The model under review builds one solid part; all positions refer to its coordinate system, in mm. Face numbers are marked on the shaded views. A direction names the side the tool comes from. Give positions to 0.01 mm unless a question says otherwise; leave off trailing zeros. Write each loop counter-clockwise with the first axis right and the second up, starting at its lowest first coordinate (ties: lowest second). Pieces come first, ordered by that corner, then holes. Notation, with made-up numbers: (76.25, 14) -> (124.25, 14) arc R20 ccw to (124.25, 22) -> close; hole circle Ø1 at (41.25, -17). An arc over 180 degrees is marked (long way). Use CSV: the item, a comma, the result in double quotes.
```python
from build123d import *

# Parameters (mm, degrees)
SKETCH1_R           = 13
SKETCH1_R_2         = 4.5
BOSS_EXTRUDE1_DEPTH = 2
SKETCH1_3_R         = 7
SKETCH1_3_R_2       = 4.5
BOSS_EXTRUDE2_DEPTH = 5
CHAMFER1_SIZE       = 1


with BuildPart() as part:
    # Sketch1 → Boss-Extrude1 (new body)
    with BuildSketch(Plane.XY):
        Circle(SKETCH1_R)
        Circle(SKETCH1_R_2, mode=Mode.SUBTRACT)
    extrude(amount=BOSS_EXTRUDE1_DEPTH)

    # Sketch1<3> → Boss-Extrude2 (add)
    with BuildSketch(Plane.XY):
        Circle(SKETCH1_3_R)
        Circle(SKETCH1_3_R_2, mode=Mode.SUBTRACT)
    extrude(amount=BOSS_EXTRUDE2_DEPTH)

    # Chamfer1
    chamfer1_edges = [part.edges().sort_by_distance(p)[0] for p in [
        (-7, 0, 5),
    ]]
    chamfer(chamfer1_edges, length=CHAMFER1_SIZE)


solid = part.part
```
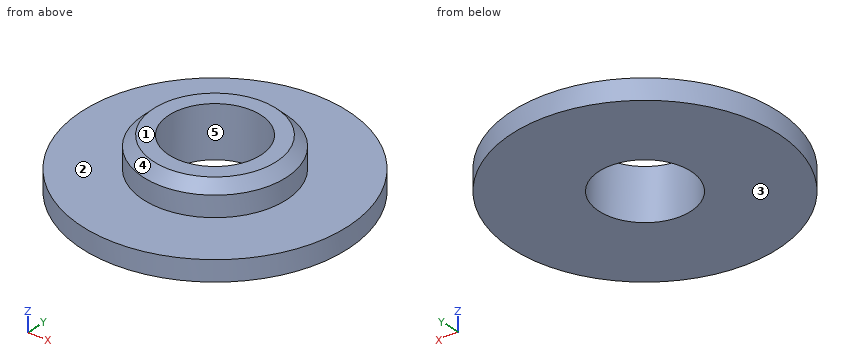
Q1. The part is to be moulded in two halves that separate along Y. For the marked faces 3, 4 and 5, say which applies: pulls with the +Y half, pulls with the -Y half, needs draft (parallel to the pull), parting line crosses it, or undercut.
Derived:
face 3,"needs draft"
face 4,"parting line crosses it"
face 5,"undercut"
Q2. Consider section A-A (x = 0). Write out the cut boundary in (y, z).
Derived:
outline,"(-13, 0) -> (-4.5, 0) -> (-4.5, 5) -> (-6, 5) -> (-7, 4) -> (-7, 2) -> (-13, 2) -> close; (4.5, 0) -> (13, 0) -> (13, 2) -> (7, 2) -> (7, 4) -> (6, 5) -> (4.5, 5) -> close"
Q3. Machinability: for the marked faces 1 and 2, which of the approach directions +Z, -Z, +X, -X, +Y, -Y give a long, thin tool a straight path to every point of the face, cutting with its end or side? Answer none if there is none.
Derived:
face 1,"+Z, +X, -X, +Y, -Y"
face 2,"+Z"
Q4. Consider section C-C (z = 3.45). Write out the cut boundary in (x, y), then the cut area to 3 significant figures.
Derived:
outline,"circle Ø14 at (0, 0); hole circle Ø9 at (0, 0)"
area,"90.3 mm2"
Q5. To check wall thickness, follow probe 1 along Y at (x, z) = (0, 2.5); probe 2 along Y at (x, z) = (0, 1.75); probe 3 along Z at (x, y) = (-5.5, -5.5). State the ranges of each line that lie inside material, in increasing order.
Derived:
probe 1,"y = -7 to -4.5, 4.5 to 7"
probe 2,"y = -13 to -4.5, 4.5 to 13"
probe 3,"z = 0 to 2"
Q6. Insertion check: pin 1 (10 mm diameter, centred on x = 10, y = -1, fed in from -Z); pin 2 (5 mm diameter, centred on x = -6.5, y = 6.5, fed in from +Z); pin 3 (5 mm diameter, centred on x = 5.5, y = 7.5, fed in from +Z); pin 4 (2 mm diameter, centred on y = -3.5, z = 1.5, fed in from -X). Each pin has a flat end and moves straight along its axis. Give the tip position at first contact, or say it passes through.
Derived:
pin 1,"stops at z = 0"
pin 2,"stops at z = 4.31"
pin 3,"stops at z = 4.2"
pin 4,"stops at x = -12.76"
Q7. Consider section D-D (x = 8.5). Write out the cut boundary in (y, z), then the cut area to 3 significant figures.
Derived:
outline,"(-9.84, 0) -> (9.84, 0) -> (9.84, 2) -> (-9.84, 2) -> close"
area,"39.3 mm2"
